For this review, take the finished solid that the model builds, in its own axes (mm). Face numbers are marked on the shaded views. A direction names the side the tool comes from. Round coordinates to 2 decimals unless told otherwise and drop trailing zeros. Order: outer loops, then holes, each group sorted by start corner. A loop starts at its lowest first (then second) coordinate and runs counter-clockwise, first axis right, second up. Notation, with made-up numbers: M 75.5,-37 L 106.5,-37 A34 cw 106.5,2 Z; hole C -27.5,61 d2. An arc over 180 degrees is marked long. Put each result on its own line as item: value.
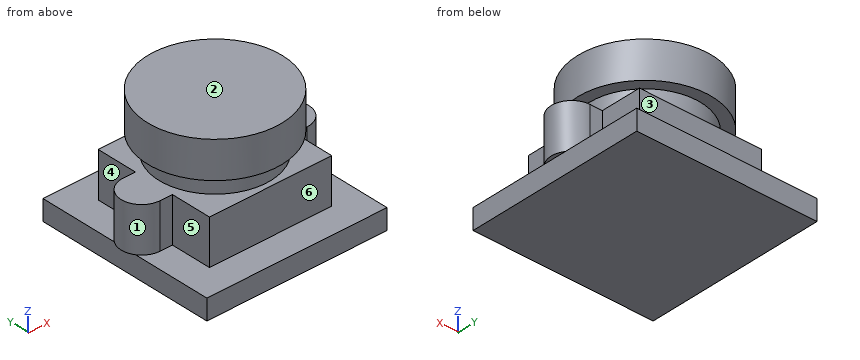
Autodesk Inventor part; units mm, degrees
ref_plane "YZ Plane" through (0, 0, 0) normal (1, 0, 0) x (0, 1, 0)
ref_plane "XZ Plane" through (0, 0, 0) normal (0, 1, 0) x (-1, 0, 0)
ref_plane "XY Plane" through (0, 0, 0) normal (0, 0, 1) x (1, 0, 0)
sketch "Sketch1" plane through (0, 0, 0) normal (0, 0, 1) x (1, 0, 0)
  line L0 (0, 0) -> (15, 0) construction
  line L1 (15, 0) -> (15, 15) construction
  line L2 (15, 15) -> (0, 15) construction
  line L3 (0, 15) -> (0, 0) construction
  circle A0 centre (-1.5, 7.5) radius 2.5 construction
  circle A1 centre (16.5, 7.5) radius 2.5 construction
  line L4 (0, 15) -> (15, 15)
  line L5 (0, 0) -> (15, 0)
  arc A2 (-1.5, 10) -> (-1.5, 5) centre (-1.5, 7.5) ccw
  arc A3 (16.5, 5) -> (16.5, 10) centre (16.5, 7.5) ccw
  line L6 (-1.5, 10) -> (0, 10)
  line L7 (-1.5, 5) -> (0, 5)
  line L8 (16.5, 10) -> (15, 10)
  line L9 (16.5, 5) -> (15, 5)
  line L10 (15, 10) -> (15, 15)
  line L11 (0, 10) -> (0, 15)
  line L12 (0, 5) -> (0, 0)
  line L13 (15, 0) -> (15, 5)
  dimension "d0" = 15
  dimension "d1" = 15
  dimension "d2" = 5
  dimension "d3" = 5
extrude "Extrusion1" add sketch "Sketch1" along normal blind 5.5
sketch "Sketch2" plane through (0, 0, 5.5) normal (0, 0, 1) x (1, 0, 0)
  line L0 (0, 5) -> (-1.5, 5)
  line L1 (7.5, 18.6806) -> (7.5, -6.0082)
  line L2 (-7.546, 7.5) -> (23.0032, 7.5)
  circle A0 centre (7.5, 7.5) radius 6.85
  dimension "d6" = 13.7
extrude "Extrusion2" add sketch "Sketch2" along normal blind 2.4
sketch "Sketch3" plane through (7.5, 7.5, 7.9) normal (0, 0, 1) x (1, 0, 0)
  circle A0 centre (0, 0) radius 6.85
  circle A1 centre (0, 0) radius 8.25
  point P0 (-7.5, -7.5)
  dimension "d9" = 16.5
extrude "Extrusion3" add sketch "Sketch3" along normal blind 4.5 contours A0 | A1
sketch "Sketch4" plane through (0, 0, 0) normal (0, 0, -1) x (-1, 0, 0)
  line L0 (-15, 0) -> (-15, 5)
  line L1 (-7.5, 18.462) -> (-7.5, -5.0214)
  line L2 (-22.4523, 7.5) -> (8.5989, 7.5)
  circle A0 centre (-7.5, 7.5) radius 11.05 construction
  line L3 (-18.55, -3.55) -> (3.55, -3.55)
  line L4 (3.55, -3.55) -> (3.55, 18.55)
  line L5 (3.55, 18.55) -> (-18.55, 18.55)
  line L6 (-18.55, 18.55) -> (-18.55, -3.55)
  dimension "d12" = 22.1
extrude "Extrusion4" add sketch "Sketch4" along normal blind 2.5
properties part number "camera"
(1) Draft analysis for pull direction Z (two halves, no side actions). For the marked faces 1, 2 and 3, state which applies: released by +Z, released by -Z, zero draft, split by the parting line, or undercut.
A:
face 1: zero draft
face 2: released by +Z
face 3: undercut
(2) Add section D-D on y = 17. Give the boundary of the cut face in (x, z), then the cut area to 4 significant figures.
A:
outline: M -3.55,-2.5 L 18.55,-2.5 L 18.55,0 L -3.55,0 Z
area: 55.25 mm2
(3) To check wall thickness, follow L1, parallel to Z at x = -1.75, y = 8.25; L2, parallel to Y at x = 2.75, z = 3.75; L3, parallel to Y at x = 7.75, z = 8.5. State the ranges of each line that lie inside material, in increasing order.
A:
L1: z = -2.5 to 5.5
L2: y = 0 to 15
L3: y = -0.75 to 15.75
(4) For the marked faces 4, 5 and 6, list the 3-axis set-ups (+Z, -Z, +X, -X, +Y, -Y) from which the entire face can be reached by the end or side of a thin tool; tool diameter is ignored.
A:
face 4: -X, +Y
face 5: -X, -Y
face 6: +X, -X, -Y
(5) Add section C-C on y = 12. Give the boundary of the cut face in (x, z).
A:
outline: M -3.55,-2.5 L 18.55,-2.5 L 18.55,0 L 15,0 L 15,5.5 L 12.66,5.5 L 12.66,7.9 L 14.41,7.9 L 14.41,12.4 L 0.59,12.4 L 0.59,7.9 L 2.34,7.9 L 2.34,5.5 L 0,5.5 L 0,0 L -3.55,0 Z
(6) Add section B-B on x = 7.5. Give the boundary of the cut face in (y, z).
A:
outline: M -3.55,-2.5 L 18.55,-2.5 L 18.55,0 L 15,0 L 15,5.5 L 14.35,5.5 L 14.35,7.9 L 15.75,7.9 L 15.75,12.4 L -0.75,12.4 L -0.75,7.9 L 0.65,7.9 L 0.65,5.5 L 0,5.5 L 0,0 L -3.55,0 Z
(7) Add section A-A on z = 0.5. Give the boundary of the cut face in (x, y).
A:
outline: M -1.5,5 L 0,5 L 0,0 L 15,0 L 15,5 L 16.5,5 A2.5 ccw 16.5,10 L 15,10 L 15,15 L 0,15 L 0,10 L -1.5,10 A2.5 ccw Z
(8) Insertion check: pin 1 Ø5 at (y, z) = (14, 4.5) entering from +X; pin 2 Ø4 at (y, z) = (2.5, 7.5) entering from +X; pin 3 Ø0.8 at (x, z) = (16, 2.5) entering from -Y; pin 4 Ø6 at (x, z) = (5, 1.5) entering from -Y. Each pin has a flat end and moves straight along its axis. Give the tip position at first contact, or say it passes through.
A:
pin 1: stops at x = 15
pin 2: stops at x = 15.17
pin 3: stops at y = 5
pin 4: stops at y = -3.55
